from build123d import *

# Parameters (mm, degrees)
SKETCH1_R           = 7
SKETCH1_R_2         = 2.5
BOSS_EXTRUDE1_DEPTH = 5
FILLET1_R           = 1
FILLET2_R           = 1


with BuildPart() as part:
    # Sketch1 → Boss-Extrude1 (new body)
    with BuildSketch(Plane(origin=(0, 0, 0), x_dir=(1, 0, 0), z_dir=(0, 1, 0))):
        Circle(SKETCH1_R)
        Circle(SKETCH1_R_2, mode=Mode.SUBTRACT)
    extrude(amount=BOSS_EXTRUDE1_DEPTH)

    # Fillet1
    fillet1_edges = [part.edges().sort_by_distance(p)[0] for p in [
        (-7, 0, 0),
        (-7, 5, 0),
    ]]
    fillet(fillet1_edges, radius=FILLET1_R)

    # Fillet2
    fillet2_edges = [part.edges().sort_by_distance(p)[0] for p in [
        (-2.5, 0, 0),
        (-2.5, 5, 0),
    ]]
    fillet(fillet2_edges, radius=FILLET2_R)


solid = part.part
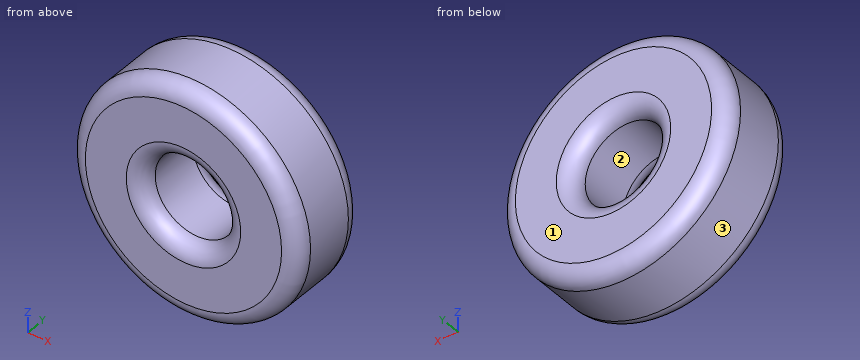
Input: part model. Units: mm. Frame: model coordinates. Face numbers are marked on the shaded views. Coordinates: 2 decimals unless noted, no trailing zeros. Order: outer loops, then holes, each group sorted by start corner. A loop starts at its lowest first (then second) coordinate and runs counter-clockwise, first axis right, second up. Notation, with made-up numbers: M 28,81 L 64,81 A19 ccw 64,118 Z; hole C 18.5,53.25 d6. An arc over 180 degrees is marked long. Answer as CSV lines item,"result".
1. First-contact query: P1, Ø3, axis at x = 3.5, y = 2, coming from the -Z side; P2, Ø1, axis at x = -5.5, y = 4, coming from the -Z side; P3, Ø4.5, axis at x = 0, z = 0, coming from the +Y side. Flat tips, straight axial feed; report the tip coordinate or a pass-through.
Reported:
P1,"z = -6.71"
P2,"z = -4.9"
P3,"through"
2. Pull-direction query (Z, two-part tool) for the marked faces 1, 2 and 3; classes: released by +Z, released by -Z, zero draft, split by the parting line, or undercut.
Reported:
face 1,"zero draft"
face 2,"undercut"
face 3,"split by the parting line"
3. Section A-A (x = 0). Return the cut outline in (y, z).
Reported:
outline,"M 0,-6 A1 ccw 1,-7 L 4,-7 A1 ccw 5,-6 L 5,-3.5 A1 ccw 4,-2.5 L 1,-2.5 A1 ccw 0,-3.5 Z; M 0,3.5 A1 ccw 1,2.5 L 4,2.5 A1 ccw 5,3.5 L 5,6 A1 ccw 4,7 L 1,7 A1 ccw 0,6 Z"
4. Section C-C (y = 0.5). Return the cut outline in (x, z).
Reported:
outline,"C 0,0 d13.73; hole C 0,0 d5.27"
5. Material intervals for line 1 (X direction, y = 3, z = 0); line 2 (Z direction, x = 2, y = 2.8), sorted ascending. Write a range as from..to.
Reported:
line 1,"-7..-2.5, 2.5..7"
line 2,"-6.71..-1.5, 1.5..6.71"
6. Section B-B (y = 2.35). Return the cut outline in (x, z).
Reported:
outline,"C 0,0 d14; hole C 0,0 d5"
